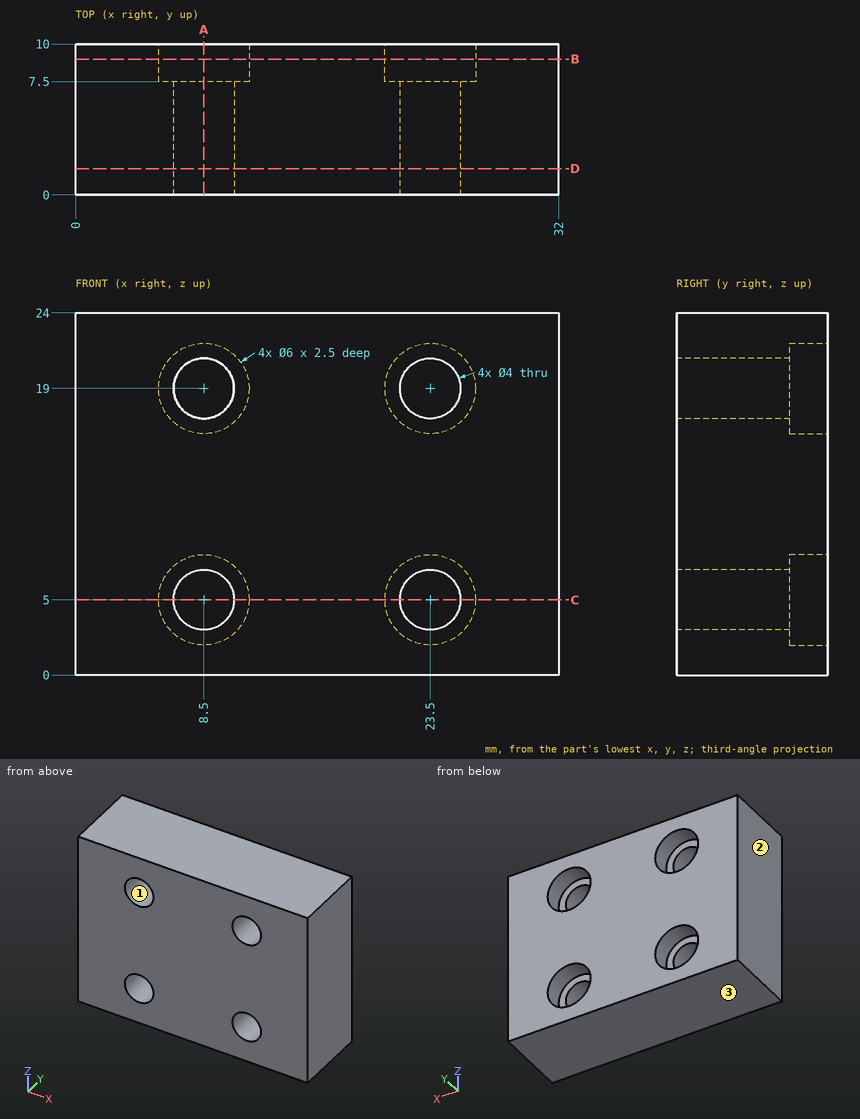
Print and shaded views of the part. All mm, measured from the part's lowest x, y and z. Coordinates: 2 decimals unless noted, no trailing zeros. Order: outer loops, then holes, each group sorted by start corner. A loop starts at its lowest first (then second) coordinate and runs counter-clockwise, first axis right, second up. Notation, with made-up numbers: (-1.75, -2) -> (32.25, -2) arc R15 cw to (32.25, 18) -> close; hole circle Ø1 at (65.5, 23.5). An arc over 180 degrees is marked (long way). Use one line per item in the form item = value. Start each with the question number.
1) Drill centre lines: L1, parallel to X at y = 8.3, z = 19; L2, parallel to Z at x = 23.5, y = 9.3; L3, parallel to X at y = 6.75, z = 17.25. Where is each one in solid material? Low to high. Write a range as [from, to].
2) Drop a flat-ended pin along its axis: pin 1 (5 mm diameter, centred on x = 23.5, z = 19, fed in from +Y). Give the stop position or say it passes through.
3) Band-saw the part on D-D on y = 1.75. Give the cut face in (x, z).
4) Band-saw the part on B-B on y = 9. Give the cut face in (x, z), then the cut area to 3 significant figures.
5) Pull direction X, two halves, no side cores. Call the marked faces 1, 2 and 3: +X half, -X half, draft (parallel to the pull), parting line (faces both ways), or undercut.
6) Band-saw the part on C-C on z = 5. Give the cut face in (x, y), then the cut area to 3 significant figures.
7) Band-saw the part on A-A on x = 8.5. Give the cut face in (y, z).
Entries:
q1.L1 = [0, 5.5], [11.5, 20.5], [26.5, 32]
q1.L2 = [0, 2], [8, 16], [22, 24]
q1.L3 = [0, 7.53], [9.47, 22.53], [24.47, 32]
q2.pin_1 = 7.5
q3.outline = (0, 0) -> (32, 0) -> (32, 24) -> (0, 24) -> close; hole circle Ø4 at (8.5, 5); hole circle Ø4 at (8.5, 19); hole circle Ø4 at (23.5, 5); hole circle Ø4 at (23.5, 19)
q4.outline = (0, 0) -> (32, 0) -> (32, 24) -> (0, 24) -> close; hole circle Ø6 at (8.5, 5); hole circle Ø6 at (8.5, 19); hole circle Ø6 at (23.5, 5); hole circle Ø6 at (23.5, 19)
q4.area = 655 mm2
q5.face_1 = undercut
q5.face_2 = -X half
q5.face_3 = draft
q6.outline = (0, 0) -> (6.5, 0) -> (6.5, 7.5) -> (5.5, 7.5) -> (5.5, 10) -> (0, 10) -> close; (10.5, 0) -> (21.5, 0) -> (21.5, 7.5) -> (20.5, 7.5) -> (20.5, 10) -> (11.5, 10) -> (11.5, 7.5) -> (10.5, 7.5) -> close; (25.5, 0) -> (32, 0) -> (32, 10) -> (26.5, 10) -> (26.5, 7.5) -> (25.5, 7.5) -> close
q6.area = 230 mm2
q7.outline = (0, 0) -> (10, 0) -> (10, 2) -> (7.5, 2) -> (7.5, 3) -> (0, 3) -> close; (0, 7) -> (7.5, 7) -> (7.5, 8) -> (10, 8) -> (10, 16) -> (7.5, 16) -> (7.5, 17) -> (0, 17) -> close; (0, 21) -> (7.5, 21) -> (7.5, 22) -> (10, 22) -> (10, 24) -> (0, 24) -> close
